from build123d import *

# Parameters (mm, degrees)
Y_KSEKLIK_EKSTR_ZYON1_DEPTH = 2.5
IZIM2_R                     = 2.5
KES_EKSTR_ZYON1_DEPTH       = 3.5
KES_EKSTR_ZYON2_DEPTH       = 3.5
IZIM5_R                     = 2.5
KES_EKSTR_ZYON3_DEPTH       = 10


with BuildPart() as part:
    # Çizim1 → Yükseklik-Ekstrüzyon1 (new body)
    with BuildSketch(Plane(origin=(0, 0, 0), x_dir=(1, 0, 0), z_dir=(0, 1, 0))):
        Polygon((0, 85), (0, 0), (73, 0), (73, 33.274387234), (49.250000664, 33.280001445), (49.262226642, 85), align=None)
    extrude(amount=Y_KSEKLIK_EKSTR_ZYON1_DEPTH)

    # Çizim2 → Kes-Ekstrüzyon1 (cut, through all)
    with BuildSketch(Plane.XZ):
        with BuildLine():
            Line((32.262752909, -52), (31.012752909, -58.015686517))
            ThreePointArc((31.012752909, -58.015686517), (33.262752909, -63), (35.512752909, -58.015686517))
            Line((35.512752909, -58.015686517), (34.262752909, -52))
            Line((34.262752909, -52), (32.262752909, -52))
        make_face()
        with Locations((33.262752909, -60)):
            Circle(IZIM2_R, mode=Mode.SUBTRACT)
        with Locations((33.262752909, -60)):
            Circle(IZIM2_R)
    extrude(amount=-KES_EKSTR_ZYON1_DEPTH, mode=Mode.SUBTRACT)

    # Çizim3 → Kes-Ekstrüzyon2 (cut, through all)
    with BuildSketch(Plane.XZ):
        with BuildLine():
            ThreePointArc((23.625155421, -47.479747819), (21.093389501, -45.218251496), (20.421796506, -41.890614625))
            ThreePointArc((20.421796506, -41.890614625), (11.442928986, -55.909121855), (14.73399817, -72.228051677))
            ThreePointArc((14.73399817, -72.228051677), (19.167411707, -73.136261128), (20.075621158, -68.70284759))
            ThreePointArc((20.075621158, -68.70284759), (17.679202056, -57.393672541), (23.625155421, -47.479747819))
        make_face()
        with BuildLine():
            ThreePointArc((23.625155421, -47.479747819), (28.709149541, -47.037034129), (31.131753414, -42.545488503))
            ThreePointArc((31.131753414, -42.545488503), (26.084801903, -37.180508616), (20.421796506, -41.890614625))
            ThreePointArc((20.421796506, -41.890614625), (22.396967687, -40.640901066), (24.492585078, -39.605781304))
            ThreePointArc((24.492585078, -39.605781304), (28.696460613, -41.281320168), (27.02092175, -45.485195703))
            ThreePointArc((27.02092175, -45.485195703), (25.260651743, -46.376256868), (23.625155421, -47.479747819))
        make_face()
        with BuildLine():
            ThreePointArc((24.492585078, -39.605781304), (22.396967687, -40.640901066), (20.421796506, -41.890614625))
            ThreePointArc((20.421796506, -41.890614625), (21.093389501, -45.218251496), (23.625155421, -47.479747819))
            ThreePointArc((23.625155421, -47.479747819), (25.260651743, -46.376256868), (27.02092175, -45.485195703))
            ThreePointArc((27.02092175, -45.485195703), (28.696460613, -41.281320168), (24.492585078, -39.605781304))
        make_face()
    extrude(amount=-KES_EKSTR_ZYON2_DEPTH, mode=Mode.SUBTRACT)

    # Çizim5 → Kes-Ekstrüzyon3 (cut)
    with BuildSketch(Plane.XZ):
        with Locations((65.19, -7.5)):
            Circle(IZIM5_R)
        with Locations((58.78, -7.5)):
            Circle(IZIM5_R)
        with Locations((52.37, -7.5)):
            Circle(IZIM5_R)
        with Locations((45.96, -7.5)):
            Circle(IZIM5_R)
        with Locations((39.55, -7.5)):
            Circle(IZIM5_R)
        with Locations((33.14, -7.5)):
            Circle(IZIM5_R)
        with Locations((26.73, -7.5)):
            Circle(IZIM5_R)
        with Locations((20.32, -7.5)):
            Circle(IZIM5_R)
        with Locations((13.91, -7.5)):
            Circle(IZIM5_R)
        with Locations((7.5, -13.59)):
            Circle(IZIM5_R)
        with Locations((7.5, -19.68)):
            Circle(IZIM5_R)
        with Locations((7.5, -25.77)):
            Circle(IZIM5_R)
        with Locations((7.5, -7.5)):
            Circle(IZIM5_R)
        with Locations((13.91, -13.59)):
            Circle(IZIM5_R)
        with Locations((20.32, -13.59)):
            Circle(IZIM5_R)
        with Locations((26.73, -13.59)):
            Circle(IZIM5_R)
        with Locations((33.14, -13.59)):
            Circle(IZIM5_R)
        with Locations((39.55, -13.59)):
            Circle(IZIM5_R)
        with Locations((45.96, -13.59)):
            Circle(IZIM5_R)
        with Locations((52.37, -13.59)):
            Circle(IZIM5_R)
        with Locations((58.78, -13.59)):
            Circle(IZIM5_R)
        with Locations((65.19, -13.59)):
            Circle(IZIM5_R)
        with Locations((13.91, -19.68)):
            Circle(IZIM5_R)
        with Locations((20.32, -19.68)):
            Circle(IZIM5_R)
        with Locations((26.73, -19.68)):
            Circle(IZIM5_R)
        with Locations((33.14, -19.68)):
            Circle(IZIM5_R)
        with Locations((39.55, -19.68)):
            Circle(IZIM5_R)
        with Locations((45.96, -19.68)):
            Circle(IZIM5_R)
        with Locations((52.37, -19.68)):
            Circle(IZIM5_R)
        with Locations((58.78, -19.68)):
            Circle(IZIM5_R)
        with Locations((65.19, -19.68)):
            Circle(IZIM5_R)
        with Locations((13.91, -25.77)):
            Circle(IZIM5_R)
        with Locations((20.32, -25.77)):
            Circle(IZIM5_R)
        with Locations((26.73, -25.77)):
            Circle(IZIM5_R)
        with Locations((33.14, -25.77)):
            Circle(IZIM5_R)
        with Locations((39.55, -25.77)):
            Circle(IZIM5_R)
        with Locations((45.96, -25.77)):
            Circle(IZIM5_R)
        with Locations((52.37, -25.77)):
            Circle(IZIM5_R)
        with Locations((58.78, -25.77)):
            Circle(IZIM5_R)
        with Locations((65.19, -25.77)):
            Circle(IZIM5_R)
    extrude(amount=-KES_EKSTR_ZYON3_DEPTH, mode=Mode.SUBTRACT)


solid = part.part
Model file for the job. Use its own axes, mm. Give positions to 0.01 mm unless a question says otherwise; leave off trailing zeros. Loops run counter-clockwise (first coordinate to the right, second up) from the corner with the lowest first, then second, coordinate; pieces in that order, holes last.
1) Flat gauge pins, fed straight in: pin 1 Ø9.5 at (x, z) = (33.26, -60) entering from +Y; pin 2 Ø4 at (x, z) = (13.91, -7.5) entering from +Y; pin 3 Ø1.2 at (x, y) = (63.5, 1.5) entering from -Z. Where does each tip first touch, or does it go through?
2) Saw through at C-C (x = 19). Write the cut outline in (y, z).
3) Saw through at D-D (z = -6). Count the separate pieces of the cut face and the enclosed holes in it, plus the area to 3 significant figures.
4) Saw through at B-B (z = -62). Write the cut outline in (x, y).
5) Wall check: line 1 (Z direction, x = 33.14, y = 2); line 2 (Z direction, x = 45.96, y = 1.9); line 3 (Z direction, x = 13, y = 2). Give the ranges that are in metal, low to high.
6) Pull direction Z, two halves, no side cores. Call faces 1 (the cylindrical face through (24.89, 1.23, -17.99)), 2 (the flat face through (28, 2.5, -53)), 3 (the flat face through (25, 1, -85)): +Z half, -Z half, draft (parallel to the pull), parting line (faces both ways), or undercut.
7) Saw through at A-A (x = 7.5). Write the cut outline in (y, z).
Answer block:
1. pin 1: stops at y = 2.5
1. pin 2: passes through
1. pin 3: stops at z = -33.28
2. outline: (0, -85) - (2.5, -85) - (2.5, -73.24) - (0, -73.24) - close; (0, -66.8) - (2.5, -66.8) - (2.5, -53.2) - (0, -53.2) - close; (0, -42.99) - (2.5, -42.99) - (2.5, -27.89) - (0, -27.89) - close; (0, -23.65) - (2.5, -23.65) - (2.5, -21.8) - (0, -21.8) - close; (0, -17.56) - (2.5, -17.56) - (2.5, -15.71) - (0, -15.71) - close; (0, -11.47) - (2.5, -11.47) - (2.5, -9.62) - (0, -9.62) - close; (0, -5.38) - (2.5, -5.38) - (2.5, 0) - (0, 0) - close
3. separate pieces: 11
3. enclosed holes: 0
3. area: 82.5 mm2
4. outline: (0, 0) - (11.15, 0) - (11.15, 2.5) - (0, 2.5) - close; (17.59, 0) - (31.03, 0) - (31.03, 2.5) - (17.59, 2.5) - close; (35.5, 0) - (49.26, 0) - (49.26, 2.5) - (35.5, 2.5) - close
5. line 1: z = -85 to -63, -52 to -28.27, -23.27 to -22.18, -17.18 to -16.09, -11.09 to -10, -5 to 0
5. line 2: z = -85 to -28.27, -23.27 to -22.18, -17.18 to -16.09, -11.09 to -10, -5 to 0
5. line 3: z = -85 to -69.07, -50.93 to -28.1, -23.44 to -22.01, -17.35 to -15.92, -11.26 to -9.83, -5.17 to 0
6. face 1: undercut
6. face 2: draft
6. face 3: -Z half
7. outline: (0, -85) - (2.5, -85) - (2.5, -28.27) - (0, -28.27) - close; (0, -23.27) - (2.5, -23.27) - (2.5, -22.18) - (0, -22.18) - close; (0, -17.18) - (2.5, -17.18) - (2.5, -16.09) - (0, -16.09) - close; (0, -11.09) - (2.5, -11.09) - (2.5, -10) - (0, -10) - close; (0, -5) - (2.5, -5) - (2.5, 0) - (0, 0) - close
